Work out the finished part from the listing and answer in its coordinate system (mm). Coordinates: 2 decimals unless noted, no trailing zeros. Write each loop counter-clockwise with the first axis right and the second up, starting at its lowest first coordinate (ties: lowest second). Pieces come first, ordered by that corner, then holes. Notation, with made-up numbers: (46, 81.5) - (89, 81.5) arc R20 cw to (89, 116.5) - close; hole circle Ø4 at (15.25, -24.75). An arc over 180 degrees is marked (long way). Use a Markdown table: item, result. Add a question column.
(1) The part is cut by section C-C, the plane x = -224. Give the vertices of the cut face in (y, z).
(2) Find the intervals of material crossed by line 1 (Y direction, x = -278.5, z = 144.78); line 2 (Y direction, x = -278, z = 144); line 3 (X direction, y = 17, z = -52.5), in increasing order. Write a range as from..to.
(3) The part is cut by section B-B, the plane z = 93. Give the vertices of the cut face in (x, y).
(4) Given pin 1 Ø7.5 at (y, z) = (43.5, 148) entering from +X; pin 2 Ø4 at (y, z) = (46, -62.5) entering from -X; pin 3 Ø3 at (y, z) = (14, 17) entering from +X, each flat-ended and moving along its own axis, determine where each tip first touches the part or whether it passes through.
(5) The part is cut by section A-A, the plane y = 13. Give the vertices of the cut face in (x, z) (3 decimals).
from build123d import *

# Parameters (mm, degrees)
BOSS_EXTRUDE1_DEPTH     = 76.2
SKETCH2_R               = 2.38125
CUT_EXTRUDE1_DEPTH      = 1
CUT_EXTRUDE1_DEPTH_BACK = 100.695


with BuildPart() as part:
    # Sketch1 → Boss-Extrude1 (new body)
    with BuildSketch(Plane(origin=(0, 0, 0), x_dir=(1, 0, 0), z_dir=(0, 1, 0))):
        Polygon((-279.4, -137.16), (-182.717603245, 153.402420415), (-179.705, 152.4), (-276.05384912, -137.16), (-276.05384912, -152.4), (-279.4, -152.4), align=None)
    extrude(amount=BOSS_EXTRUDE1_DEPTH)

    # Sketch2 → Cut-Extrude1 (cut, two sides)
    with BuildSketch(Plane.ZY.offset(279.4)) as cut_extrude1_sk:
        with Locations((144.78, 38.1)):
            Circle(SKETCH2_R)
    extrude(amount=CUT_EXTRUDE1_DEPTH, mode=Mode.SUBTRACT)
    extrude(cut_extrude1_sk.sketch, amount=-CUT_EXTRUDE1_DEPTH_BACK, mode=Mode.SUBTRACT)


solid = part.part
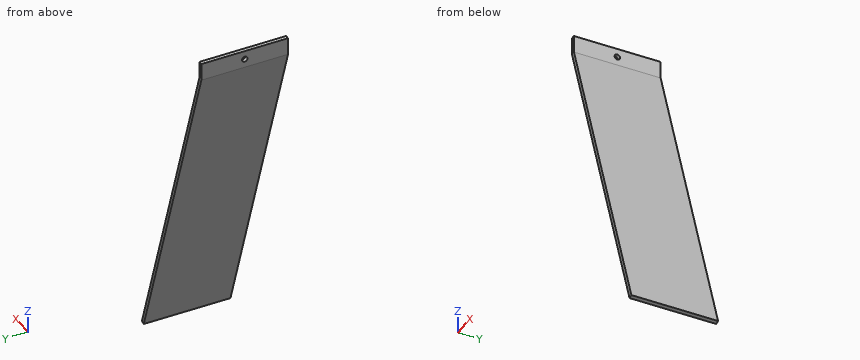
Model answer:
| question | item | result |
|---|---|---|
| 1 | outline | (0, -29.34) - (76.2, -29.34) - (76.2, -19.28) - (0, -19.28) - close |
| 2 | line 1 | 0..35.72, 40.48..76.2 |
| 2 | line 2 | 0..35.85, 40.35..76.2 |
| 2 | line 3 | -216.29..-212.95 |
| 3 | outline | (-264.71, 0) - (-261.36, 0) - (-261.36, 76.2) - (-264.71, 76.2) - close |
| 4 | pin 1 | x = -276.05 |
| 4 | pin 2 | x = -213.63 |
| 4 | pin 3 | x = -235.57 |
| 5 | outline | (-279.4, 137.16) - (-182.718, -153.402) - (-179.705, -152.4) - (-276.054, 137.16) - (-276.054, 152.4) - (-279.4, 152.4) - close |
